Could you check a few things on this model? Use its own coordinates, in mm. A direction names the side the tool comes from. Coordinates: 2 decimals unless noted, no trailing zeros. Order: outer loops, then holes, each group sorted by start corner. A loop starts at its lowest first (then second) coordinate and runs counter-clockwise, first axis right, second up. Notation, with made-up numbers: (-39.75, 35.25) - (10.25, 35.25) arc R17 ccw to (10.25, 59.25) - close; hole circle Ø1 at (-0.75, 26.25). An arc over 180 degrees is marked (long way). One line per item, written item: value. Start each with the question number.
from build123d import *

# Parameters (mm, degrees)
SKETCH1_W            = 55
SKETCH1_H            = 25.7
BOSS_EXTRUDE1_DEPTH  = 3
SKETCH2_W            = 41
SKETCH2_H            = 20.7
CUT_EXTRUDE1_DEPTH   = 31.502008131
SKETCH3_R            = 2.1
CUT_EXTRUDE2_DEPTH   = 31.502008131
SKETCH4_W            = 41
SKETCH4_H            = 2.5
BOSS_EXTRUDE2_DEPTH  = 20
CUT_EXTRUDE3_DEPTH   = 0.375
FILLET1_R            = 5
SKETCH6_W            = 41
SKETCH6_H            = 2.5
BOSS_EXTRUDE3_DEPTH  = 7
SKETCH7_W            = 20
SKETCH7_H            = 3
BOSS_EXTRUDE4_DEPTH  = 12.9
SKETCH8_R            = 2.1
CUT_EXTRUDE4_DEPTH   = 47.349892125
FILLET2_R            = 5
FILLET2_OF_MIRROR5_R = 5


with BuildPart() as part:
    # Sketch1 → Boss-Extrude1 (new body)
    with BuildSketch(Plane(origin=(0, 0, 0), x_dir=(1, 0, 0), z_dir=(0, 1, 0))):
        Rectangle(SKETCH1_W, SKETCH1_H)
    extrude(amount=BOSS_EXTRUDE1_DEPTH)

    # Sketch2 → Cut-Extrude1 (cut, through all)
    with BuildSketch(Plane(origin=(0, 3, 0), x_dir=(1, 0, 0), z_dir=(0, 1, 0))):
        Rectangle(SKETCH2_W, SKETCH2_H)
    extrude(amount=-CUT_EXTRUDE1_DEPTH, mode=Mode.SUBTRACT)

    # Sketch3 → Cut-Extrude2 (cut, through all)
    with BuildSketch(Plane(origin=(0, 3, 0), x_dir=(1, 0, 0), z_dir=(0, 1, 0))):
        with Locations(Location((24.35, 5.85, 0), (0, 0, 270))):
            Circle(SKETCH3_R)
        with Locations(Location((24.35, -5.85, 0), (0, 0, 270))):
            Circle(SKETCH3_R)
    cut_extrude2 = extrude(amount=-CUT_EXTRUDE2_DEPTH, mode=Mode.SUBTRACT)

    # Mirror1: Cut-Extrude2 across plane
    add(cut_extrude2.mirror(Plane(origin=(0, 0, 0), x_dir=(0, 0, 1), z_dir=(1, 0, 0))), mode=Mode.SUBTRACT)

    # Sketch4 → Boss-Extrude2 (add)
    with BuildSketch(Plane(origin=(0, 3, 0), x_dir=(1, 0, 0), z_dir=(0, 1, 0))):
        with Locations((0, 11.6)):
            Rectangle(SKETCH4_W, SKETCH4_H)
        with Locations((0, -11.6)):
            Rectangle(SKETCH4_W, SKETCH4_H)
    extrude(amount=BOSS_EXTRUDE2_DEPTH)

    # Sketch5 → Cut-Extrude3 (cut, symmetric)
    with BuildSketch(Plane.XY):
        Polygon((20.5, 1), (20.5, 3), (28.245966692, 3), align=None)
    cut_extrude3 = extrude(amount=CUT_EXTRUDE3_DEPTH, both=True, mode=Mode.SUBTRACT)

    # Mirror2: Cut-Extrude3 across plane
    add(cut_extrude3.mirror(Plane(origin=(0, 0, 0), x_dir=(0, 0, 1), z_dir=(1, 0, 0))), mode=Mode.SUBTRACT)

    # Fillet1
    fillet1_edges = [part.edges().sort_by_distance(p)[0] for p in [
        (-27.5, 1.5, -12.85),
        (27.5, 1.5, -12.85),
        (27.5, 1.5, 12.85),
        (-27.5, 1.5, 12.85),
    ]]
    fillet(fillet1_edges, radius=FILLET1_R)

    # Sketch6 → Boss-Extrude3 (add)
    with BuildSketch(Plane.XZ):
        with Locations((0, 11.6)):
            Rectangle(SKETCH6_W, SKETCH6_H)
        with Locations((0, -11.6)):
            Rectangle(SKETCH6_W, SKETCH6_H)
    extrude(amount=BOSS_EXTRUDE3_DEPTH)

    # Sketch7 → Boss-Extrude4 (add)
    with BuildSketch(Plane.XY.offset(12.85)):
        with Locations((0, -5.5)):
            Rectangle(SKETCH7_W, SKETCH7_H)
    boss_extrude4 = extrude(amount=BOSS_EXTRUDE4_DEPTH)

    # Sketch8 → Cut-Extrude4 (cut, through all)
    with BuildSketch(Plane(origin=(0, -4, 0), x_dir=(1, 0, 0), z_dir=(0, 1, 0))):
        with Locations(Location((0, -20.75, 0), (0, 0, 270))):
            Circle(SKETCH8_R)
    cut_extrude4 = extrude(amount=-CUT_EXTRUDE4_DEPTH, mode=Mode.SUBTRACT)

    # Fillet2
    fillet2_edges = [part.edges().sort_by_distance(p)[0] for p in [
        (-10, -5.5, 25.75),
        (10, -5.5, 25.75),
    ]]
    fillet(fillet2_edges, radius=FILLET2_R)

    # Mirror5: Boss-Extrude4, Cut-Extrude4 across plane
    add(boss_extrude4.mirror(Plane.XY))
    add(cut_extrude4.mirror(Plane.XY), mode=Mode.SUBTRACT)

    # Fillet2 of Mirror5
    fillet2_of_mirror5_edges = [part.edges().sort_by_distance(p)[0] for p in [
        (-10, -5.5, -25.75),
        (10, -5.5, -25.75),
    ]]
    fillet(fillet2_of_mirror5_edges, radius=FILLET2_OF_MIRROR5_R)


solid = part.part
Q1. I want a section at C-C on z = 5.85. Please give me the cut outline in (x, y), then the cut area to 3 significant figures.
Q2. Which directions (+Z, -Z, +X, -X, +Y, -Y) give clear straight access to the entire face, cutting with the end or side of a thin tool? Please do faces 5 (the flat face through (-10, -6, -17)), 6 (the flat face through (-10, -6, 17)), 7 (the flat face through (0, -4, -18)), 8 (the flat face through (-24, 0, 0)), 9 (the flat face through (-23, 2, 0.375)).
Q3. We'd pull the mould along Z, two halves only. Please class faces 1 (the flat face through (0, -5, -25.75)), 2 (the flat face through (-23, 2, -0.375)), 3 (the flat face through (27.5, 1, 0)), 4 (the cylindrical face through (-8.57, -5.48, 24.25)): +Z half, -Z half, draft (parallel to the pull), parting line (faces both ways), or undercut.
Q4. I'm going to push flat-ended pins straight in: pin 1 (2 mm diameter, centred on y = -2.5, z = 11, fed in from -X); pin 2 (7.5 mm diameter, centred on x = -22.5, z = -5.5, fed in from -Y); pin 3 (5 mm diameter, centred on x = 10.5, y = 10.5, fed in from -Z); pin 4 (2.5 mm diameter, centred on x = 0, z = 20.75, fed in from +Y). Where does each tip first touch, or does it pass through?
Q5. I want a section at A-A on z = -1.5. Please give me the cut outline in (x, y).
Q6. I want a section at B-B on x = 0. Please give me the cut outline in (y, z), then the cut area to 3 significant figures.
Q7. I want a section at D-D on y = 5.5. Please give me the cut outline in (x, z).
Q8. If I drill on L1, parallel to X at y = 1.85, z = -5.85; L2, parallel to Z at x = -2.5, y = 17.5; L3, parallel to X at y = -5.25, z = 20.75, over which ranges is the centre line in solid material (lowest first)?
Values follow:
1. outline: (-27.5, 0) - (-26.45, 0) - (-26.45, 3) - (-27.5, 3) - close; (-22.25, 0) - (-20.5, 0) - (-20.5, 3) - (-22.25, 3) - close; (20.5, 0) - (22.25, 0) - (22.25, 3) - (20.5, 3) - close; (26.45, 0) - (27.5, 0) - (27.5, 3) - (26.45, 3) - close
1. area: 16.8 mm^2
2. face 5: -Z, -X, +Y, -Y
2. face 6: +Z, -X, +Y, -Y
2. face 7: -Z, +X, -X, +Y
2. face 8: +Z, -Z, -X, -Y
2. face 9: +Y
3. face 1: -Z half
3. face 2: undercut
3. face 3: draft
3. face 4: +Z half
4. pin 1: stops at x = -20.5
4. pin 2: stops at y = 0
4. pin 3: stops at z = -12.85
4. pin 4: passes through
5. outline: (-27.5, 0) - (-20.5, 0) - (-20.5, 3) - (-27.5, 3) - close; (20.5, 0) - (27.5, 0) - (27.5, 3) - (20.5, 3) - close
6. outline: (-7, -25.75) - (-4, -25.75) - (-4, -22.85) - (-7, -22.85) - close; (-7, -18.65) - (-4, -18.65) - (-4, -12.85) - (23, -12.85) - (23, -10.35) - (-7, -10.35) - close; (-7, 10.35) - (23, 10.35) - (23, 12.85) - (-4, 12.85) - (-4, 18.65) - (-7, 18.65) - close; (-7, 22.85) - (-4, 22.85) - (-4, 25.75) - (-7, 25.75) - close
6. area: 202 mm^2
7. outline: (-20.5, -12.85) - (20.5, -12.85) - (20.5, -10.35) - (-20.5, -10.35) - close; (-20.5, 10.35) - (20.5, 10.35) - (20.5, 12.85) - (-20.5, 12.85) - close
8. L1: x = -27.5 to -26.45, -22.25 to -20.5, 20.5 to 22.25, 26.45 to 27.5
8. L2: z = -12.85 to -10.35, 10.35 to 12.85
8. L3: x = -10 to -2.1, 2.1 to 10
